Could you check a few things on this drawing? It's one solid part, dimensions in mm from its lowest x, y, z. A direction names the side the tool comes from. Round coordinates to 2 decimals unless told otherwise and drop trailing zeros. Write each loop counter-clockwise with the first axis right and the second up, starting at its lowest first coordinate (ties: lowest second). Pieces come first, ordered by that corner, then holes. Notation, with made-up numbers: (24.5, 19.5) -> (79.5, 19.5) arc R25 ccw to (79.5, 47.5) -> close; hole circle Ø11 at (-37, 71). An arc over 180 degrees is marked (long way). Put each result on its own line as item: value. Start each with the question number.
1) I want a section at A-A, the plane z = 8.25. List the corners of the cut face in (x, y) for me.
2) If I drill on line 1 along Y through (x, z) = (41.5, 4.5); line 2 along X through (y, z) = (2, 2); line 3 along Z through (x, y) = (16, 1.25), over which ranges is the centre line in solid material (lowest first)? Write a range as [from, to].
3) We'd pull the mould along Z, two halves only. Please class the marked faces 3, 4, 5 and 6: released by +Z, released by -Z, zero draft, split by the parting line, or undercut.
4) I want a section at B-B, the plane x = 41.5. List the corners of the cut face in (y, z) for me.
5) I want a section at C-C, the plane z = 3. List the corners of the cut face in (x, y) for me.
6) I want a section at D-D, the plane y = 5. Give the number of separate pieces and of enclosed holes in the cut face, then the cut area to 3 significant figures.
7) Which directions (+Z, -Z, +X, -X, +Y, -Y) give clear straight access to the entire face, cutting with the end or side of a thin tool? Please do the marked faces 1 and 2.
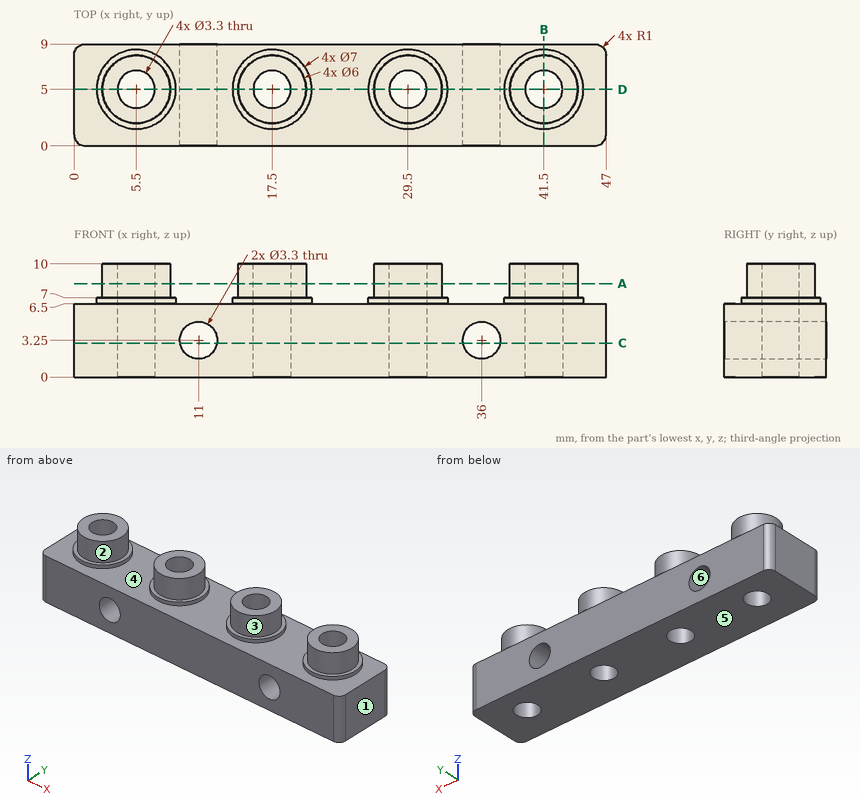
Findings:
1. outline: circle Ø6 at (5.5, 5); circle Ø6 at (17.5, 5); circle Ø6 at (29.5, 5); circle Ø6 at (41.5, 5); hole circle Ø3.3 at (5.5, 5); hole circle Ø3.3 at (17.5, 5); hole circle Ø3.3 at (29.5, 5); hole circle Ø3.3 at (41.5, 5)
2. line 1: y = [0, 3.35], [6.65, 9]
2. line 2: x = [0, 9.92], [12.08, 34.92], [37.08, 47]
2. line 3: z = [0, 6.5]
3. face 3: zero draft
3. face 4: released by +Z
3. face 5: released by -Z
3. face 6: undercut
4. outline: (0, 0) -> (3.35, 0) -> (3.35, 10) -> (2, 10) -> (2, 7) -> (1.5, 7) -> (1.5, 6.5) -> (0, 6.5) -> close; (6.65, 0) -> (9, 0) -> (9, 6.5) -> (8.5, 6.5) -> (8.5, 7) -> (8, 7) -> (8, 10) -> (6.65, 10) -> close
5. outline: (0, 1) arc R1 ccw to (1, 0) -> (9.37, 0) -> (9.37, 9) -> (1, 9) arc R1 ccw to (0, 8) -> close; (12.63, 0) -> (34.37, 0) -> (34.37, 9) -> (12.63, 9) -> close; (37.63, 0) -> (46, 0) arc R1 ccw to (47, 1) -> (47, 8) arc R1 ccw to (46, 9) -> (37.63, 9) -> close; hole circle Ø3.3 at (5.5, 5); hole circle Ø3.3 at (17.5, 5); hole circle Ø3.3 at (29.5, 5); hole circle Ø3.3 at (41.5, 5)
6. separate pieces: 5
6. enclosed holes: 2
6. area: 242 mm2
7. face 1: +Z, -Z, +X, +Y, -Y
7. face 2: +Z
